The listing builds one solid part. Answer for the finished solid, in the listing's coordinates (mm). Face numbers are marked on the shaded views. A direction names the side the tool comes from. Give positions to 0.01 mm unless a question says otherwise; leave off trailing zeros. Order: outer loops, then holes, each group sorted by start corner. A loop starts at its lowest first (then second) coordinate and runs counter-clockwise, first axis right, second up. Notation, with made-up numbers: (55.5, 27) - (114.5, 27) arc R32 cw to (114.5, 56) - close; hole circle Ø7 at (63.5, -12.5). An arc over 180 degrees is marked (long way). Answer as a JSON object with one key per item and string values. Group by question number.
Q1. For the marked faces 1 and 2, determine the directions among +Z, -Z, +X, -X, +Y, -Y from which every point of the face is accessible in a straight line to the end or side of a thin tool.
Q2. Given pin 1 (1 mm diameter, centred on x = 10.5, y = -216, fed in from -Z); pin 2 (8 mm diameter, centred on y = -185.5, z = -9, fed in from -X); pin 3 (6 mm diameter, centred on x = 8, y = -211, fed in from +Z), each flat-ended and moving along its own axis, determine where each tip first touches the part or whether it passes through.
Q3. Consider line 1 (X direction, y = -33, z = 1); line 2 (Y direction, x = 6, z = 16). Determine where each line is inside the solid, lowest interval first.
Q4. A cutting plane is placed at A-A, the plane y = -3. Give the vertices of the cut face in (x, z).
from build123d import *

# Parameters (mm, degrees)
BOSS_EXTRUDE1_DEPTH = 20
SKETCH2_OUTSIDE_W   = 123.112
SKETCH2_OUTSIDE_H   = 117.698
SKETCH2_OUTSIDE_R   = 17.5
CUT_EXTRUDE1_DEPTH  = 20
CUT_EXTRUDE1_TAPER  = 60
SKETCH3_R           = 13
BOSS_EXTRUDE2_DEPTH = 300


with BuildPart() as part:
    # Sketch1 → Boss-Extrude1 (new body)
    with BuildSketch(Plane(origin=(0, 0, 0), x_dir=(1, 0, 0), z_dir=(0, 1, 0))):
        Polygon((-10.103629711, -17.5), (10.103629711, -17.5), (20.207259422, 0), (10.103629711, 17.5), (-10.103629711, 17.5), (-20.207259422, 0), align=None)
    extrude(amount=BOSS_EXTRUDE1_DEPTH)

    # Sketch2 outside → Cut-Extrude1 (cut)
    with BuildSketch(Plane(origin=(0, 20, 0), x_dir=(1, 0, 0), z_dir=(0, 1, 0))):
        Rectangle(SKETCH2_OUTSIDE_W, SKETCH2_OUTSIDE_H)
        Circle(SKETCH2_OUTSIDE_R, mode=Mode.SUBTRACT)
    extrude(amount=-CUT_EXTRUDE1_DEPTH, taper=CUT_EXTRUDE1_TAPER, mode=Mode.SUBTRACT)

    # Sketch3 → Boss-Extrude2 (add)
    with BuildSketch(Plane.XZ):
        Circle(SKETCH3_R)
    extrude(amount=BOSS_EXTRUDE2_DEPTH)


solid = part.part
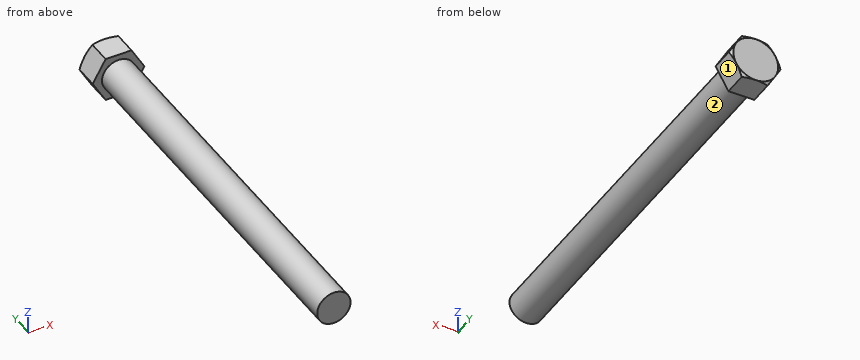
Reply:
{
 "1": {"face 1": "-Z, +X, +Y, -Y", "face 2": "-Y"},
 "2": {"pin 1": "stops at z = -8.31", "pin 2": "stops at x = -12", "pin 3": "stops at z = 12"},
 "3": {"line 1": "x = -12.96 to 12.96", "line 2": "y = 0 to 20"},
 "4": {"outline": "circle Ø26 at (0, 0)"}
}
